Design review of the part shown in the three views and the two pictorial views. Dimensions are in mm from the part's minimum x, y and z. A direction names the side the tool comes from. Give positions to 0.01 mm unless a question says otherwise; leave off trailing zeros. Loops run counter-clockwise (first coordinate to the right, second up) from the corner with the lowest first, then second, coordinate; pieces in that order, holes last.
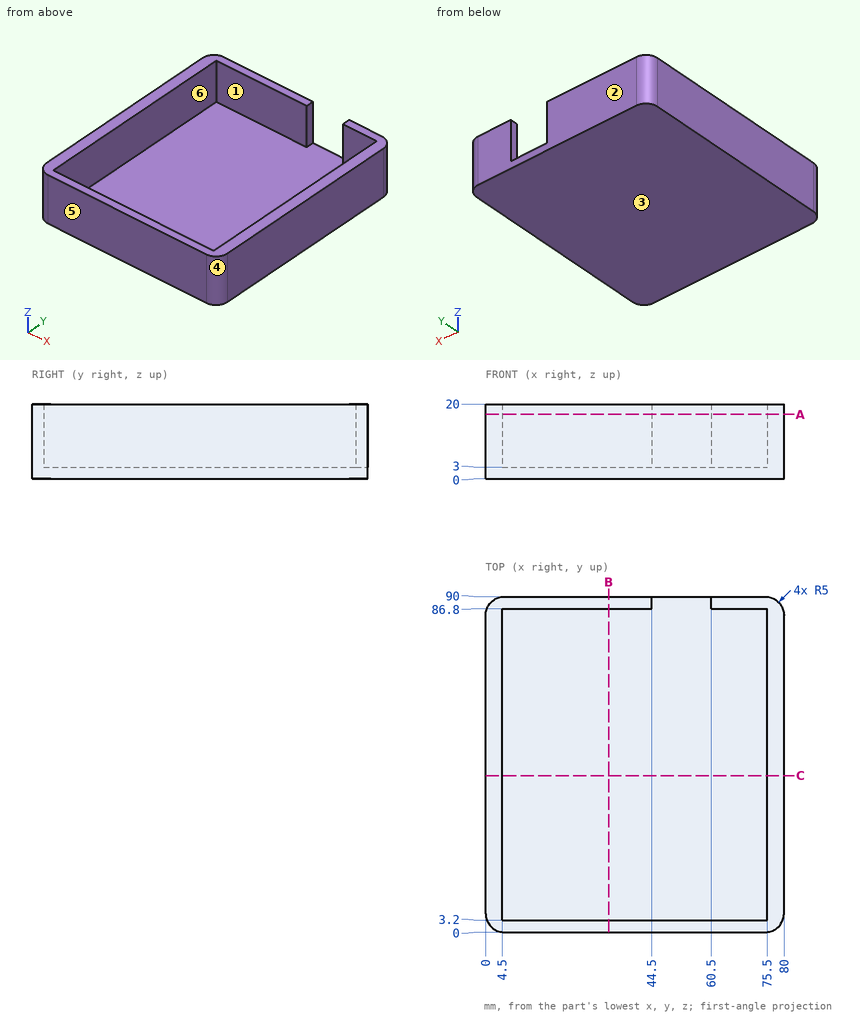
Q1. Mouldability with a two-part tool opening along Y and no side actions: class the marked faces 1, 2, 3 and 4 as +Y half, -Y half, draft (parallel to the pull), parting line (faces both ways), or undercut.
Answers:
face 1: undercut
face 2: +Y half
face 3: draft
face 4: -Y half
Q2. Consider section C-C on y = 42. Give the boundary of the cut face in (x, z), plus the area to 3 significant figures.
Answers:
outline: (0, 0) - (80, 0) - (80, 20) - (75.5, 20) - (75.5, 3) - (4.5, 3) - (4.5, 20) - (0, 20) - close
area: 393 mm2
Q3. For probe 1 along X at (y, z) = (16.5, 17); probe 2 along Y at (x, z) = (67.5, 11.5); probe 3 along Y at (x, z) = (53, 10.25), list the stretches that pass through material, from the lowest coordinate up.
Answers:
probe 1: x = 0 to 4.5, 75.5 to 80
probe 2: y = 0 to 3.2, 86.8 to 90
probe 3: y = 0 to 3.2
Q4. Machinability: for the marked faces 5 and 6, which of the approach directions +Z, -Z, +X, -X, +Y, -Y give a long, thin tool a straight path to every point of the face, cutting with its end or side? Answer none if there is none.
Answers:
face 5: +Z, -Z, +X, -X, -Y
face 6: +Z
Q5. For pin 1 Ø2.5 at (y, z) = (89, 12.5) entering from -X; pin 2 Ø3.5 at (y, z) = (88, 12.5) entering from +X, all flat-tipped, find the tip position at first contact; note any pin that passes through.
Answers:
pin 1: stops at x = 0.82
pin 2: stops at x = 79.84
Q6. Consider section A-A on z = 17.25. Give the boundary of the cut face in (x, y), plus the area to 3 significant figures.
Answers:
outline: (0, 5) arc R5 ccw to (5, 0) - (75, 0) arc R5 ccw to (80, 5) - (80, 85) arc R5 ccw to (75, 90) - (60.5, 90) - (60.5, 86.8) - (75.5, 86.8) - (75.5, 3.2) - (4.5, 3.2) - (4.5, 86.8) - (44.5, 86.8) - (44.5, 90) - (5, 90) arc R5 ccw to (0, 85) - close
area: 1,190 mm2
Q7. Consider section B-B on x = 33. Give the boundary of the cut face in (y, z).
Answers:
outline: (0, 0) - (90, 0) - (90, 20) - (86.8, 20) - (86.8, 3) - (3.2, 3) - (3.2, 20) - (0, 20) - close
